Can you work these out from the model? Positions are in its coordinate system, mm. Coordinates: 2 decimals unless noted, no trailing zeros. Order: outer loops, then holes, each group sorted by start corner. A loop starts at its lowest first (then second) coordinate and runs counter-clockwise, first axis right, second up. Notation, with made-up numbers: (58.25, -6) - (81.25, -6) arc R25 cw to (81.25, 25) - close; hole circle Ø7 at (18, 29). An arc over 180 degrees is marked (long way). Use a Markdown table: item, result. Add a question column.
(1) I want a section at C-C (z = -76.2). List the corners of the cut face in (x, y) for me (3 decimals), and give its area (3 significant figures).
(2) I want a section at D-D (y = 0). List the corners of the cut face in (x, z) for me (3 decimals), and give its area (3 significant figures).
(3) If I drill on L1, parallel to Y at x = -0.25, z = -57.5 (1 decimal); L2, parallel to Z at x = -0.25, y = 17.78; L3, parallel to Z at x = -1.25, y = 25.5, over which ranges is the centre line in solid material (lowest first)? Write a range as [from, to].
(4) For pin 1 Ø3 at (x, y) = (-0.5, -0.5) entering from -Z; pin 2 Ø3 at (x, z) = (1.5, 122) entering from -Y; pin 3 Ø1.9 at (x, z) = (0.5, 116.5) entering from +Y, each with a flat end and sliding along its axis, tell me the tip position at first contact or that it passes through.
(5) I want a section at B-B (z = -39). List the corners of the cut face in (x, y) for me (1 decimal).
```python
from build123d import *

# Parameters (mm, degrees)
F0_R     = 3.81
F1_DEPTH = 3.175


# Not quite as in the source:
# - ends of sketch curves that miss each other by under 0.0002 mm in the source are joined


with BuildPart() as f1:
    # F0 (on Right) → F1 (new body, symmetric)
    with BuildSketch(Plane.YZ):
        Polygon((28.575, -63.5), (23.8125, -63.5), (3.175, -63.5), (3.175, -88.9), (28.575, -88.9), align=None)
        with Locations((17.78, -76.2)):
            Circle(F0_R, mode=Mode.SUBTRACT)
        with BuildLine():
            Line((3.175, -63.5), (23.8125, -63.5))
            Line((23.8125, -63.5), (23.8125, 57.15))
            ThreePointArc((23.8125, 57.15), (21.9533763667, 61.6393796296), (17.4646167058, 63.4999996472))
            Line((17.4646167058, 63.4999996472), (17.4625, 63.5))
            Line((17.4625, 63.5), (11.1139111112, 63.5))
            Line((11.1139111112, 63.5), (11.124494366, 158.7492930333))
            ThreePointArc((11.124494366, 158.7492930333), (9.2648719104, 163.2398771909), (4.7744944052, 165.0999985889))
            Line((4.7744944052, 165.0999985889), (-4.7498, 165.0999985889))
            ThreePointArc((-4.7498, 165.0999985889), (-9.2399280605, 163.2401266494), (-11.0998, 158.7499985889))
            Line((-11.0998, 158.7499985889), (-11.0998, 63.5))
            Line((-11.0998, 63.5), (-17.4498, 63.5))
            Line((-17.4498, 63.5), (-17.4625, 63.5))
            ThreePointArc((-17.4625, 63.5), (-21.9526280605, 61.6401280605), (-23.8125, 57.15))
            Line((-23.8125, 57.15), (-23.8125, -63.5))
            Line((-23.8125, -63.5), (-3.175, -63.5))
            Line((-3.175, -63.5), (-3.175, 63.5))
            Line((-3.175, 63.5), (3.175, 63.5))
            Line((3.175, 63.5), (3.175, -63.5))
        make_face()
    extrude(amount=F1_DEPTH, both=True)


solid = f1.part
```
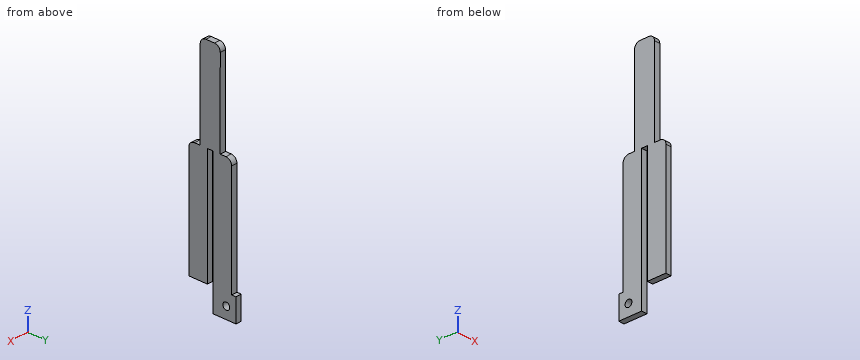
Answers follow:
| question | item | result |
|---|---|---|
| 1 | outline | (-3.175, 3.175) - (3.175, 3.175) - (3.175, 13.97) - (-3.175, 13.97) - close; (-3.175, 21.59) - (3.175, 21.59) - (3.175, 28.575) - (-3.175, 28.575) - close |
| 1 | area | 113 mm² |
| 2 | outline | (-3.175, 63.5) - (3.175, 63.5) - (3.175, 165.1) - (-3.175, 165.1) - close |
| 2 | area | 645 mm² |
| 3 | L1 | y = [-23.8, -3.2], [3.2, 23.8] |
| 3 | L2 | z = [-88.9, -80.01], [-72.39, 63.49] |
| 3 | L3 | z = [-88.9, -63.5] |
| 4 | pin 1 | stops at z = 63.5 |
| 4 | pin 2 | stops at y = -11.1 |
| 4 | pin 3 | stops at y = 11.12 |
| 5 | outline | (-3.2, -23.8) - (3.2, -23.8) - (3.2, -3.2) - (-3.2, -3.2) - close; (-3.2, 3.2) - (3.2, 3.2) - (3.2, 23.8) - (-3.2, 23.8) - close |
